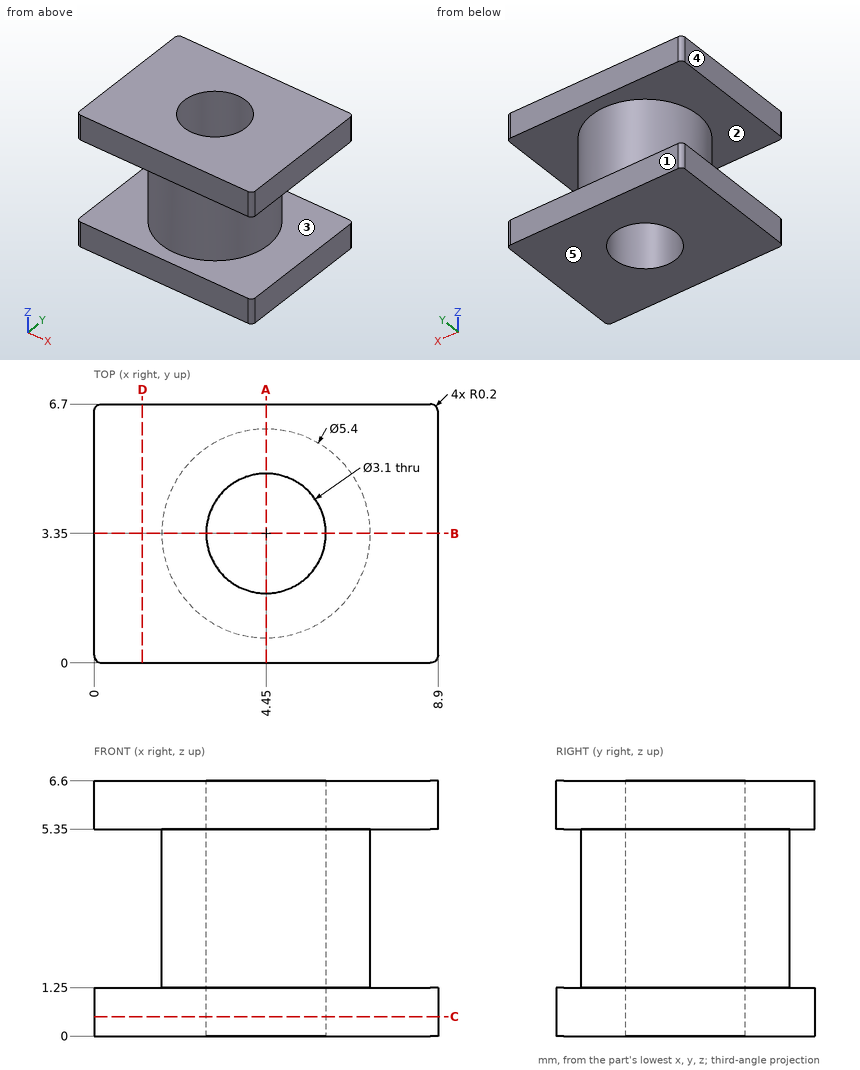
Here's the drawing with two shaded views (mm, measured from the low corner). I have some questions. A direction names the side the tool comes from. Give positions to 0.01 mm unless a question says otherwise; leave off trailing zeros. Loops run counter-clockwise (first coordinate to the right, second up) from the corner with the lowest first, then second, coordinate; pieces in that order, holes last. Notation, with made-up numbers: (81, 70.5) - (102, 70.5) arc R9 ccw to (102, 82.5) - close; hole circle Ø4 at (-5, 77.25). An arc over 180 degrees is marked (long way). Answer in a Markdown table with one row per item. Add a question column.
Q1. If we section it at D-D (x = 1.25): List the corners of the cut face in (y, z) for me, plus the area to 4 significant figures.
Q2. For pin 1 (2 mm diameter, centred on x = 5, y = 4, fed in from -Z); pin 2 (2 mm diameter, centred on y = 3.5, z = 3, fed in from +X), each with a flat end and sliding along its axis, tell me the tip position at first contact or that it passes through.
Q3. If we section it at C-C (z = 0.5): List the corners of the cut face in (x, y) for me.
Q4. We'd pull the mould along Z, two halves only. Please class the marked faces 3, 4 and 5: +Z half, -Z half, draft (parallel to the pull), parting line (faces both ways), or undercut.
Q5. Which directions (+Z, -Z, +X, -X, +Y, -Y) give clear straight access to the entire face, cutting with the end or side of a thin tool? Please do the marked faces 1 and 2.
Q6. If we section it at B-B (y = 3.35): List the corners of the cut face in (x, z) for me, plus the area to 3 significant figures.
Q7. If we section it at A-A (x = 4.45): List the corners of the cut face in (y, z) for me, plus the area to 3 significant figures.
Q8. Please list where these lines run through material, in increasing order: L1, parallel to Z at x = 7.75, y = 2.5; L2, parallel to Y at x = 4.45, z = 3.25; L3, parallel to X at y = 2.75, z = 2. Write a range as from..to.
The answers:
| question | item | result |
|---|---|---|
| 1 | outline | (0, 0) - (6.7, 0) - (6.7, 1.25) - (0, 1.25) - close; (0, 5.35) - (6.7, 5.35) - (6.7, 6.6) - (0, 6.6) - close |
| 1 | area | 16.75 mm^2 |
| 2 | pin 1 | stops at z = 0 |
| 2 | pin 2 | stops at x = 7.15 |
| 3 | outline | (0, 0.2) arc R0.2 ccw to (0.2, 0) - (8.7, 0) arc R0.2 ccw to (8.9, 0.2) - (8.9, 6.5) arc R0.2 ccw to (8.7, 6.7) - (0.2, 6.7) arc R0.2 ccw to (0, 6.5) - close; hole circle Ø3.1 at (4.45, 3.35) |
| 4 | face 3 | undercut |
| 4 | face 4 | draft |
| 4 | face 5 | -Z half |
| 5 | face 1 | +Z, -Z, +X, -X, +Y |
| 5 | face 2 | none |
| 6 | outline | (0, 0) - (2.9, 0) - (2.9, 6.6) - (0, 6.6) - (0, 5.35) - (1.75, 5.35) - (1.75, 1.25) - (0, 1.25) - close; (6, 0) - (8.9, 0) - (8.9, 1.25) - (7.15, 1.25) - (7.15, 5.35) - (8.9, 5.35) - (8.9, 6.6) - (6, 6.6) - close |
| 6 | area | 23.9 mm^2 |
| 7 | outline | (0, 0) - (1.8, 0) - (1.8, 6.6) - (0, 6.6) - (0, 5.35) - (0.65, 5.35) - (0.65, 1.25) - (0, 1.25) - close; (4.9, 0) - (6.7, 0) - (6.7, 1.25) - (6.05, 1.25) - (6.05, 5.35) - (6.7, 5.35) - (6.7, 6.6) - (4.9, 6.6) - close |
| 7 | area | 18.4 mm^2 |
| 8 | L1 | z = 0..1.25, 5.35..6.6 |
| 8 | L2 | y = 0.65..1.8, 4.9..6.05 |
| 8 | L3 | x = 1.82..3.02, 5.88..7.08 |
